Check sheet for the modelled part. Datum: model origin and axes. Units: mm. Face numbers are marked on the shaded views. Round coordinates to 2 decimals unless told otherwise and drop trailing zeros. Loops run counter-clockwise (first coordinate to the right, second up) from the corner with the lowest first, then second, coordinate; pieces in that order, holes last. Notation, with made-up numbers: (29.5, 0) - (78.5, 0) arc R9 cw to (78.5, 11) - close; hole circle Ø2 at (-13, 14). An arc over 180 degrees is marked (long way). Put each result on its own line as item: value. Start each with the question number.
Item 1: Gauge pin test, flat end, axial feed: pin 1 Ø10 at (x, y) = (10, -15.5) entering from -Z. Record the tip position at first contact, or that the pin passes through.
Item 2: Section check A-A, the plane z = 2.8. Give the number of separate pieces and of enclosed holes in the cut face, and give its area (3 significant figures).
Item 3: Section check B-B, the plane x = -0.25. Record the cut outline in (y, z) (3 decimals), and give its area (3 significant figures).
Item 4: Draft check along Z on the marked faces 1 and 2. Enter one of: pulls with the +Z half, pulls with the -Z half, needs draft (parallel to the pull), parting line crosses it, or undercut.
Item 5: Material ranges on line 1 along Y through (x, z) = (3, 2.35) (3 decimals); line 2 along Y through (x, z) = (4, 3.4) (3 decimals); line 3 along X through (y, z) = (-59, 2.8), recorded low to high.
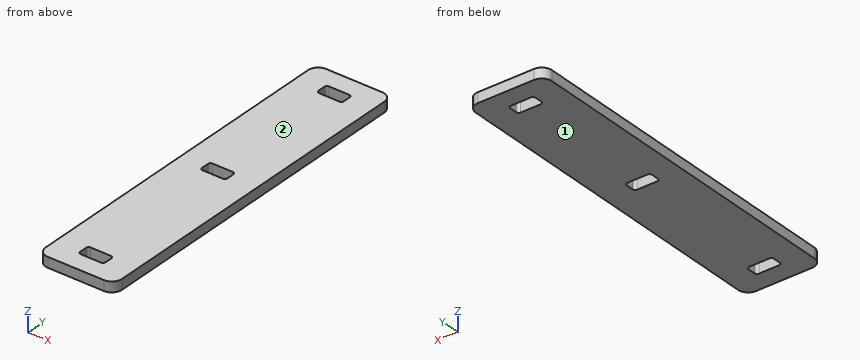
from build123d import *

# Parameters (mm, degrees)
BOSS_EXTRU_1_DEPTH      = 4
ENL_V_MAT_EXTRU_1_DEPTH = 72.617785675


with BuildPart() as part:
    # Esquisse1 → Boss.-Extru.1 (new body)
    with BuildSketch(Plane.XY):
        with BuildLine():
            Line((-11, -69.915), (11, -69.915))
            ThreePointArc((11, -69.915), (13.828427125, -68.743427125), (15, -65.915))
            Line((15, -65.915), (15, 65.915))
            ThreePointArc((15, 65.915), (13.828427125, 68.743427125), (11, 69.915))
            Line((11, 69.915), (-11, 69.915))
            ThreePointArc((-11, 69.915), (-13.828427125, 68.743427125), (-15, 65.915))
            Line((-15, 65.915), (-15, -65.915))
            ThreePointArc((-15, -65.915), (-13.828427125, -68.743427125), (-11, -69.915))
        make_face()
    extrude(amount=BOSS_EXTRU_1_DEPTH)

    # Esquisse2 → Enlèv. mat.-Extru.1 (cut, through all)
    with BuildSketch(Plane.XY.offset(4)):
        with BuildLine():
            Line((-4, -57.415), (4, -57.415))
            ThreePointArc((4, -57.415), (4.707106781, -57.707893219), (5, -58.415))
            Line((5, -58.415), (5, -61.415))
            ThreePointArc((5, -61.415), (4.707106781, -62.122106781), (4, -62.415))
            Line((4, -62.415), (-4, -62.415))
            ThreePointArc((-4, -62.415), (-4.707106781, -62.122106781), (-5, -61.415))
            Line((-5, -61.415), (-5, -58.415))
            ThreePointArc((-5, -58.415), (-4.707106781, -57.707893219), (-4, -57.415))
        make_face()
        with BuildLine():
            Line((-4, 62.415), (4, 62.415))
            ThreePointArc((4, 62.415), (4.707106781, 62.122106781), (5, 61.415))
            Line((5, 61.415), (5, 58.415))
            ThreePointArc((5, 58.415), (4.707106781, 57.707893219), (4, 57.415))
            Line((4, 57.415), (-4, 57.415))
            ThreePointArc((-4, 57.415), (-4.707106781, 57.707893219), (-5, 58.415))
            Line((-5, 58.415), (-5, 61.415))
            ThreePointArc((-5, 61.415), (-4.707106781, 62.122106781), (-4, 62.415))
        make_face()
        with BuildLine():
            Line((-4.587622439, 4.585), (3.412377561, 4.585))
            ThreePointArc((3.412377561, 4.585), (4.119484342, 4.292106781), (4.412377561, 3.585))
            Line((4.412377561, 3.585), (4.412377561, 0.585))
            ThreePointArc((4.412377561, 0.585), (4.119484342, -0.122106781), (3.412377561, -0.415))
            Line((3.412377561, -0.415), (-4.587622439, -0.415))
            ThreePointArc((-4.587622439, -0.415), (-5.29472922, -0.122106781), (-5.587622439, 0.585))
            Line((-5.587622439, 0.585), (-5.587622439, 3.585))
            ThreePointArc((-5.587622439, 3.585), (-5.29472922, 4.292106781), (-4.587622439, 4.585))
        make_face()
    extrude(amount=-ENL_V_MAT_EXTRU_1_DEPTH, mode=Mode.SUBTRACT)


solid = part.part
Check result:
1. pin 1: z = 0
2. separate pieces: 1
2. enclosed holes: 3
2. area: 4,030 mm²
3. outline: (-69.915, 0) - (-62.415, 0) - (-62.415, 4) - (-69.915, 4) - close; (-57.415, 0) - (-0.415, 0) - (-0.415, 4) - (-57.415, 4) - close; (4.585, 0) - (57.415, 0) - (57.415, 4) - (4.585, 4) - close; (62.415, 0) - (69.915, 0) - (69.915, 4) - (62.415, 4) - close
3. area: 499 mm²
4. face 1: pulls with the -Z half
4. face 2: pulls with the +Z half
5. line 1: -69.915 to -62.415, -57.415 to -0.415, 4.585 to 57.415, 62.415 to 69.915
5. line 2: -69.915 to -62.415, -57.415 to -0.224, 4.394 to 57.415, 62.415 to 69.915
5. line 3: -15 to -5, 5 to 15
